Part print with two shaded views. Sizes in mm from the minimum x, y, z corner. Coordinates: 2 decimals unless noted, no trailing zeros. Write each loop counter-clockwise with the first axis right and the second up, starting at its lowest first coordinate (ties: lowest second). Pieces come first, ordered by that corner, then holes. Notation, with made-up numbers: (37.5, 49) - (83.5, 49) arc R15 ccw to (83.5, 68) - close; hole circle Ø3 at (62, 49.25). An arc over 180 degrees is marked (long way). Answer in a Markdown table with one row per item. Add a question column.
Q1. Band-saw the part on A-A (x = 3.5). List the corners of the cut face in (y, z).
Q2. Drill centre lines: line 1 along Z through (x, y) = (7.5, 6); line 2 along Y through (x, z) = (49, 92); line 3 along Y through (x, z) = (24, 8). Where is each one in solid material? Low to high. Write a range as from..to.
Q3. Band-saw the part on B-B (y = 21.5). List the corners of the cut face in (x, z).
Q4. Pin check, flat tip, straight feed: pin 1 (2 mm diameter, centred on y = 9.5, z = 70, fed in from -X). Stop position of the tip, or through.
Q5. Band-saw the part on C-C (z = 49.5). List the corners of the cut face in (x, y), and give its area (3 significant figures).
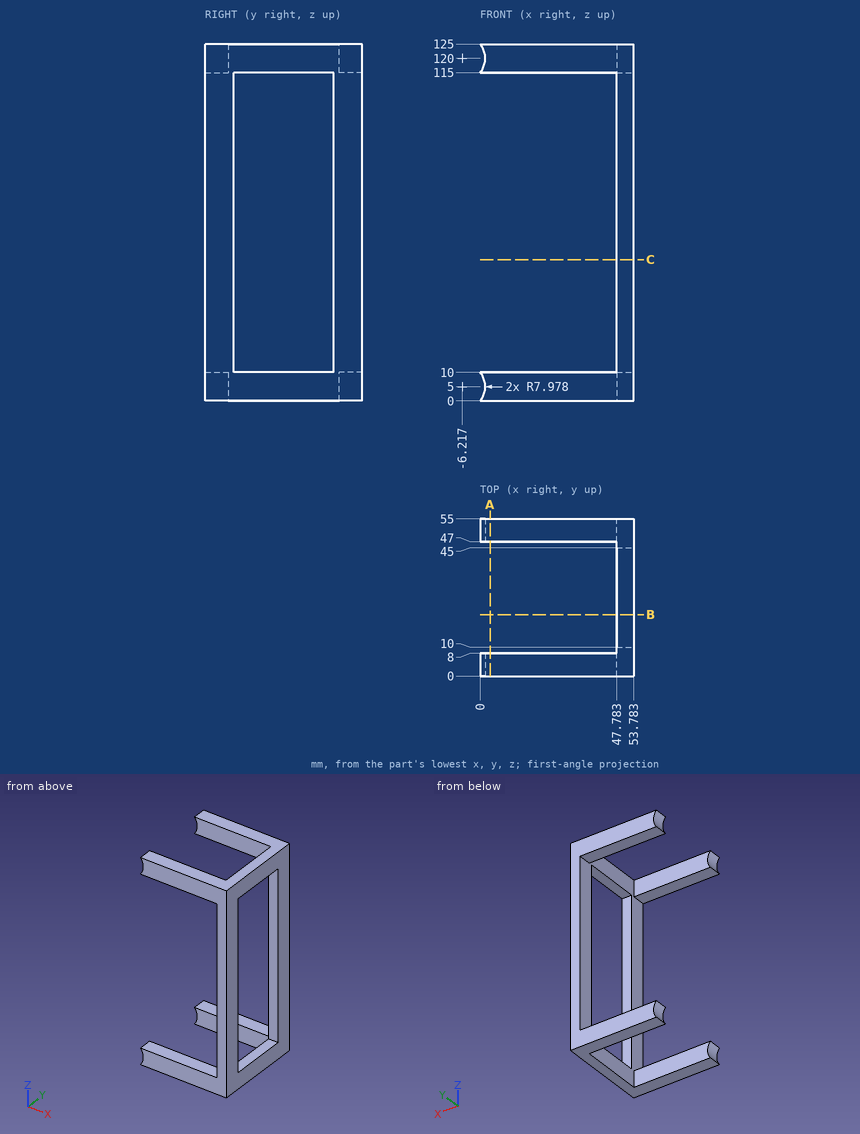
Checked values:
| question | item | result |
|---|---|---|
| 1 | outline | (0, 0) - (8, 0) - (8, 10) - (0, 10) - close; (0, 115) - (8, 115) - (8, 125) - (0, 125) - close; (47, 0) - (55, 0) - (55, 10) - (47, 10) - close; (47, 115) - (55, 115) - (55, 125) - (47, 125) - close |
| 2 | line 1 | z = 0..10, 115..125 |
| 2 | line 2 | y = 0..10, 45..55 |
| 2 | line 3 | y = 0..8, 47..55 |
| 3 | outline | (47.78, 0) - (53.78, 0) - (53.78, 10) - (47.78, 10) - close; (47.78, 115) - (53.78, 115) - (53.78, 125) - (47.78, 125) - close |
| 4 | pin 1 | stops at x = 47.78 |
| 5 | outline | (47.78, 0) - (53.78, 0) - (53.78, 10) - (47.78, 10) - close; (47.78, 45) - (53.78, 45) - (53.78, 55) - (47.78, 55) - close |
| 5 | area | 120 mm² |
